Geometry: final body of the model. Coordinates: model frame, mm. Face numbers are marked on the shaded views. A direction names the side the tool comes from. Round coordinates to 2 decimals unless told otherwise and drop trailing zeros. Loops run counter-clockwise (first coordinate to the right, second up) from the corner with the lowest first, then second, coordinate; pieces in that order, holes last. Notation, with made-up numbers: (-28.75, 28.5) -> (-18.75, 28.5) arc R20 ccw to (-18.75, 46.5) -> close; hole circle Ø11 at (-31, 39.5). An arc over 180 degrees is marked (long way). Answer in a Markdown table with one row per item.
Autodesk Inventor part; units mm, degrees
ref_plane "YZ Plane" through (0, 0, 0) normal (1, 0, 0) x (0, 1, 0)
ref_plane "XZ Plane" through (0, 0, 0) normal (0, 1, 0) x (-1, 0, 0)
ref_plane "XY Plane" through (0, 0, 0) normal (0, 0, 1) x (1, 0, 0)
sketch "Sketch1" plane through (0, 0, 0) normal (0, 1, 0) x (-1, 0, 0)
  line L0 (0, 0) -> (40, 0)
  line L1 (40, 0) -> (40, -60)
  line L2 (40, -60) -> (0, -60)
  line L3 (0, -60) -> (0, 0)
  dimension "d0" = 40
  dimension "d1" = 60
extrude "Plate1" add sketch "Sketch1" along normal blind 0.5
sketch "Sketch2" plane through (-39.5, 0, 0) normal (-1, 0, 0) x (0, -1, 0)
  line L0 (0, -60) -> (0, 0)
  line L1 (0, 0) -> (-47, 0)
  line L2 (-47, 0) -> (-47, -60)
  line L3 (-47, -60) -> (0, -60)
edge flange "Flange1" height 47 angle 90 thickness 0.5 bend radius 0.5 thickness toward (-1, 0, 0) relief tear relief width 0.5 relief depth 0.25 corner gap 0.5 corner form 0 edges at (-40, 0.5, -30) (0, 0.5, -30) wall of the first edge with corners at (-39.5, 0, -60) (-39.5, 0, 0) (-39.5, 47, 0) (-39.5, 47, -60)
bend "Bend1"
corner "Corner1"
sketch "Sketch4" plane through (-40, 47, -60) normal (-1, 0, 0) x (0, 0, 1)
  circle A0 centre (42, -18) radius 11
  line L0 (60, 0) -> (60, -46)
  line L1 (0, 0) -> (60, 0)
  point P0 (60, -47)
  dimension "d14" = 22
  dimension "d15" = 18
  dimension "d16" = 18
extrude "Cut1" cut sketch "Sketch4" against normal up to surface (40 mm away)
chamfer "Corner Chamfer1" distance 32 angle 45 2 edges at (-0.25, 47, -60) (-39.75, 47, -60)
fillet "Corner Round1" radius 15 4 edges at (-39.75, 47, -28) (-39.75, 47, 0) (-0.25, 47, 0) (-0.25, 47, -28)
sketch "Sketch5" plane through (0, 0.5, 0) normal (0, 1, 0) x (1, 0, 0)
  circle A0 centre (-20, 12) radius 4.15
  circle A1 centre (-20, 48) radius 4.15
  line L0 (-1, 0) -> (-39, 0)
  line L1 (-39, 60) -> (-1, 60)
  point P0 (0, 0)
  point P1 (-20, 0)
  dimension "d23" = 8.3
  dimension "d24" = 8.3
  dimension "d25" = 12
  dimension "d26" = 12
extrude "Cut2" cut sketch "Sketch5" against normal up to surface (0.5 mm away)
equation "\"d17\" = Thickness"
equation "\"d27\" = Thickness"
equation "\"d2\" = Thickness"
equation "\"d3\" = BendReliefWidth"
equation "\"d4\" = BendReliefDepth"
equation "\"d5\" = MinimumRemnant"
equation "\"d6\" = TransitionRadius"
equation "\"d9\" = BendRadius"
equation "\"d10\" = CornerReliefSize"
equation "\"d11\" = GapSize"
equation "\"d12\" = JacobiRadiusSize"
equation "\"BendRadius\" = Thickness"
equation "\"BendReliefWidth\" = Thickness"
equation "\"BendReliefDepth\" = 0.5 * Thickness"
equation "\"CornerReliefSize\" = 4 * Thickness"
equation "\"MinimumRemnant\" = 2 * Thickness"
equation "\"TransitionRadius\" = BendRadius"
equation "\"JacobiRadiusSize\" = BendRadius"
equation "\"GapSize\" = Thickness"
equation "\"A_width\" = 46"
equation "\"A_joint_diameter\" = 16"
equation "\"A_B_spacing\" = 2"
equation "\"A_joint_tolerance\" = 3"
equation "\"l___________\" = 0"
equation "\"l__________\" = 0"
equation "\"l_________\" = 0"
equation "\"rivet_diameter\" = 3.35"
equation "\"plate_thickness\" = 3"
equation "\"l________\" = 0"
equation "\"L_Piston_Top\" = 25"
equation "\"L_Piston_Bottom\" = 21"
properties part number "profile_mount-1"
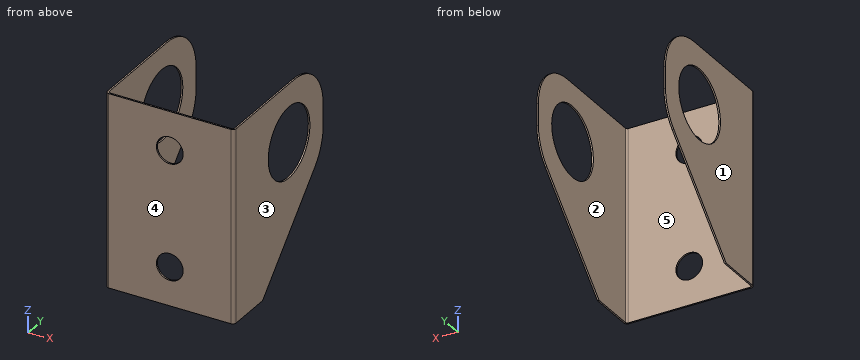
Item 1: Line query: probe 1 along Z at (x, y) = (-20, 0.1); probe 2 along X at (y, z) = (3.5, -54.5); probe 3 along Y at (x, z) = (-29, -10). Output: solid intervals per line, ascending. Write a range as [from, to].
Answer:
| item | result |
|---|---|
| probe 1 | z = [-60, -52.15], [-43.85, -16.15], [-7.85, 0] |
| probe 2 | x = [-40, -39.5], [-0.5, 0] |
| probe 3 | y = [0, 0.5] |
Item 2: Pin query (flat end, axial travel): pin 1 Ø7.5 at (x, z) = (-20, -48) entering from +Y; pin 2 Ø19 at (x, z) = (-25.5, -26.5) entering from +Y. Return the tip coordinate at first contact, or that it passes through.
Answer:
| item | result |
|---|---|
| pin 1 | passes through |
| pin 2 | stops at y = 0.5 |
Item 3: Cut plane B-B (y = 13.5). Output: boundary loops of the cut face in (x, z).
Answer:
| item | result |
|---|---|
| outline | (-40, -60) -> (-39.5, -60) -> (-39.5, 0) -> (-40, 0) -> close; (-0.5, -60) -> (0, -60) -> (0, 0) -> (-0.5, 0) -> close |
Item 4: Cut plane A-A (z = -48). Output: boundary loops of the cut face in (x, y), then the cut area to 3 significant figures.
Answer:
| item | result |
|---|---|
| outline | (-40, 1) arc R1 ccw to (-39, 0) -> (-24.15, 0) -> (-24.15, 0.5) -> (-39, 0.5) arc R0.5 cw to (-39.5, 1) -> (-39.5, 27) -> (-40, 27) -> close; (-15.85, 0) -> (-1, 0) arc R1 ccw to (0, 1) -> (0, 27) -> (-0.5, 27) -> (-0.5, 1) arc R0.5 cw to (-1, 0.5) -> (-15.85, 0.5) -> close |
| area | 42.0 mm² |
Item 5: Cut plane C-C (x = -20). Output: boundary loops of the cut face in (y, z), then the cut area to 3 significant figures.
Answer:
| item | result |
|---|---|
| outline | (0, -60) -> (0.5, -60) -> (0.5, -52.15) -> (0, -52.15) -> close; (0, -43.85) -> (0.5, -43.85) -> (0.5, -16.15) -> (0, -16.15) -> close; (0, -7.85) -> (0.5, -7.85) -> (0.5, 0) -> (0, 0) -> close |
| area | 21.7 mm² |
Item 6: Reachability of the marked faces 1 and 2 from +Z, -Z, +X, -X, +Y, -Y: full face, straight path, thin tool, end or side. Return the list, or none.
Answer:
| item | result |
|---|---|
| face 1 | +Z, -Z, -X, +Y, -Y |
| face 2 | +Z, -Z, +Y |
Item 7: Cut plane D-D (y = 29). Output: boundary loops of the cut face in (x, z).
Answer:
| item | result |
|---|---|
| outline | (-40, -46) -> (-39.5, -46) -> (-39.5, -29) -> (-40, -29) -> close; (-40, -7) -> (-39.5, -7) -> (-39.5, 0) -> (-40, 0) -> close; (-0.5, -46) -> (0, -46) -> (0, -29) -> (-0.5, -29) -> close; (-0.5, -7) -> (0, -7) -> (0, 0) -> (-0.5, 0) -> close |
Item 8: Draft query along X for the marked faces 3, 4 and 5. Return one class per face: pulls with the +X half, pulls with the -X half, needs draft (parallel to the pull), parting line crosses it, or undercut.
Answer:
| item | result |
|---|---|
| face 3 | pulls with the +X half |
| face 4 | needs draft |
| face 5 | undercut |
